Autodesk Inventor part; units mm, degrees
ref_plane "YZ Plane" through (0, 0, 0) normal (1, 0, 0) x (0, 1, 0)
ref_plane "XZ Plane" through (0, 0, 0) normal (0, 1, 0) x (-1, 0, 0)
ref_plane "XY Plane" through (0, 0, 0) normal (0, 0, 1) x (1, 0, 0)
ref_plane "Work Plane5" through (0, 3, 0) normal (0, 1, 0) x (1, 0, 0)
sketch "Sketch45" plane through (0, 3, 0) normal (0, 1, 0) x (1, 0, 0)
  line L0 (35, -20) -> (-3, -20)
  line L1 (-3, -20) -> (-3, 20)
  line L2 (-3, 20) -> (35, 20)
  line L3 (35, 20) -> (35, -20)
  point P0 (0, 0)
  dimension "d142" = 38
  dimension "d143" = 40
extrude "Extrusion34" add sketch "Sketch45" along normal blind 30
ref_plane "Work Plane2" through (0, 0, 0) normal (0, -1, 0) x (1, 0, 0)
sketch "Sketch47" plane through (0, 0, 0) normal (0, -1, 0) x (1, 0, 0)
  circle A0 centre (16, 0) radius 18
  point P0 (0, 0)
  dimension "d146" = 36
extrude "Extrusion35" cut sketch "Sketch47" against normal blind 30 draft -15
ref_plane "Work Plane1" through (0, 3, 0) normal (0, 1, 0) x (1, 0, 0)
sketch "Sketch74" plane through (0, 33, 0) normal (0, 1, 0) x (1, 0, 0)
  circle A0 centre (20, 0) radius 1.15
  point P0 (0, 0)
  dimension "d210" = 2.3
extrude "Extrusion51" cut sketch "Sketch74" against normal blind 10
sketch "Sketch77" plane through (0, 3, 0) normal (0, -1, 0) x (1, 0, 0)
  circle A0 centre (16, 0) radius 17.5
  point P0 (0, 0)
  dimension "d219" = 35
sketch "Sketch78" plane through (0, 3, 0) normal (0, -1, 0) x (1, 0, 0)
  line L0 (45, -30) -> (-13, -30)
  line L1 (-13, -30) -> (-13, 30)
  line L2 (-13, 30) -> (45, 30)
  line L3 (45, 30) -> (45, -30)
  line L4 (45, -30) -> (-13, 30) construction
  line L5 (-13, -30) -> (45, 30) construction
  point P0 (0, 0)
  point P1 (16, 0)
  dimension "d220" = 58
  dimension "d221" = 60
extrude "Extrusion53" add sketch "Sketch78" against normal blind 3
extrude "Extrusion54" cut sketch "Sketch77" against normal blind 3
sketch "Sketch81" plane through (0, 3, 0) normal (0, -1, 0) x (1, 0, 0)
  circle A0 centre (33.5, -25) radius 2.7
  line L0 (-13, -30) -> (45, -30)
  line L1 (45, -30) -> (45, 30)
  circle A1 centre (16, -25) radius 2.7
  circle A2 centre (-1.5, -25) radius 2.7
  circle A3 centre (-6.5, -8) radius 2.7
  circle A4 centre (-6.5, 8) radius 2.7
  circle A5 centre (-1.5, 25) radius 2.7
  circle A6 centre (16, 25) radius 2.7
  circle A7 centre (33.5, 25) radius 2.7
  point P0 (0, 0)
  dimension "mag_D" = 5.4
  dimension "d232" = 5
  dimension "d233" = 11.5
  dimension "d234" = 5.4
  dimension "d235" = 17.5
  dimension "d236" = 5.4
  dimension "d237" = 17.5
  dimension "d238" = 5.4
  dimension "d239" = 5
  dimension "d240" = 17
  dimension "d241" = 5.4
  dimension "d242" = 16
  dimension "d243" = 5.4
  dimension "d244" = 17
  dimension "d245" = 5.4
  dimension "d246" = 17.5
  dimension "d247" = 5.4
  dimension "d248" = 17.5
  dimension "d249" = 5
extrude "Extrusion56" cut sketch "Sketch81" against normal blind 30
equation "\"d234\" = mag_D"
equation "\"d236\" = mag_D"
equation "\"d237\" = d235"
equation "\"d238\" = mag_D"
equation "\"d241\" = mag_D"
equation "\"d243\" = mag_D"
equation "\"d244\" = d240"
equation "\"d245\" = mag_D"
equation "\"d246\" = d235"
equation "\"d247\" = mag_D"
equation "\"d248\" = d235"
equation "\"d249\" = d239"
properties part number "liquid_port_v02"
Verification items for the finished model (mm, model axes). A direction names the side the tool comes from. Round coordinates to 2 decimals unless told otherwise and drop trailing zeros. Write each loop counter-clockwise with the first axis right and the second up, starting at its lowest first coordinate (ties: lowest second). Pieces come first, ordered by that corner, then holes. Notation, with made-up numbers: (15.5, 45) - (19.5, 45) arc R18 cw to (19.5, 58) - close; hole circle Ø1 at (40, -15). An arc over 180 degrees is marked (long way). Answer as a JSON object with one key per item and string values. Group by question number.
Q1. Mould release check, pull along X, two halves, no side actions. Record for faces 5 (the conical face through (27.554, 20.499, -4.79)), 6 (the flat face through (16, 33, 0)), 7 (the cylindrical face through (33.149, 4.479, -22.323)), 8 (the flat face through (45, 4, 0)): released by +X, released by -X, zero draft, split by the parting line, or undercut.
Q2. Section check B-B, the plane x = -6.5. Enter the section's corners in (y, z), plus the area to 3 significant figures.
Q3. Section check C-C, the plane z = 25. Enter the section's corners in (x, y), plus the area to 3 significant figures.
Q4. Tool access check on faces 1 (the cylindrical face through (18.85, 31.52, -0.05)), 2 (the flat face through (16, 19, 20)), 3 (the flat face through (-3, 19, 0)), 4 (the flat face through (16, 30, 0)). Record the directions out of +Z, -Z, +X, -X, +Y, -Y that give a thin tool (end or side, any length) a straight path to the whole face; none if there is none.
Q5. Section check A-A, the plane z = 0. Enter the section's corners in (x, y).
Q6. Go/stop test with flat-tipped pins: pin 1 Ø13.5 at (y, z) = (24.5, -8.5) entering from -X; pin 2 Ø5 at (x, z) = (-1.5, -25) entering from -Y; pin 3 Ø8 at (x, y) = (13.5, 24.5) entering from -Z; pin 4 Ø1.5 at (x, z) = (0.5, -21) entering from +Y. Record where each tip stops, or that it passes through.
Q7. Thickness scan on line 1 (Z direction, x = 16, y = 4.05); line 2 (Z direction, x = 20, y = 31.3); line 3 (X direction, y = 32.1, z = 0). Record the ranges inside material, lowest first.
Q8. Section check D-D, the plane y = 10. Enter the section's corners in (x, z).
Found:
{
 "1": {"face 5": "undercut", "face 6": "zero draft", "face 7": "undercut", "face 8": "released by +X"},
 "2": {"outline": "(3, -30) - (6, -30) - (6, -10.7) - (3, -10.7) - close; (3, -5.3) - (6, -5.3) - (6, 5.3) - (3, 5.3) - close; (3, 10.7) - (6, 10.7) - (6, 30) - (3, 30) - close", "area": "148 mm^2"},
 "3": {"outline": "(-13, 3) - (-4.2, 3) - (-4.2, 6) - (-13, 6) - close; (1.2, 3) - (13.3, 3) - (13.3, 6) - (1.2, 6) - close; (18.7, 3) - (30.8, 3) - (30.8, 6) - (18.7, 6) - close; (36.2, 3) - (45, 3) - (45, 6) - (36.2, 6) - close", "area": "125 mm^2"},
 "4": {"face 1": "+Y, -Y", "face 2": "+Z, +X, -X, +Y", "face 3": "+Z, -Z, -X, +Y", "face 4": "-Y"},
 "5": {"outline": "(-13, 3) - (-1.5, 3) - (-1.5, 6) - (-0.39, 6) - (6.04, 30) - (18.85, 30) - (18.85, 33) - (-3, 33) - (-3, 6) - (-13, 6) - close; (21.15, 30) - (25.96, 30) - (32.39, 6) - (33.5, 6) - (33.5, 3) - (45, 3) - (45, 6) - (35, 6) - (35, 33) - (21.15, 33) - close"},
 "6": {"pin 1": "stops at x = -3", "pin 2": "passes through", "pin 3": "stops at z = -20", "pin 4": "stops at y = 6"},
 "7": {"line 1": "z = -30 to -27.7, -22.3 to -17.5, 17.5 to 22.3, 27.7 to 30", "line 2": "z = -20 to -1.15, 1.15 to 20", "line 3": "x = -3 to 18.85, 21.15 to 35"},
 "8": {"outline": "(-3, -20) - (35, -20) - (35, 20) - (-3, 20) - close; hole circle Ø30.64 at (16, 0)"}
}
